Verification items for the finished model (mm, model axes). A direction names the side the tool comes from. Coordinates: 2 decimals unless noted, no trailing zeros. Order: outer loops, then holes, each group sorted by start corner. A loop starts at its lowest first (then second) coordinate and runs counter-clockwise, first axis right, second up. Notation, with made-up numbers: M 11.25,-38 L 61.25,-38 A31 ccw 61.25,-13 Z; hole C -32,-10 d9. An arc over 180 degrees is marked long. Return JSON: item names as keys, results as strings. Group by question number.
1. Section check C-C, the plane x = 0.5. Record the cut outline in (y, z).
2. Section check A-A, the plane x = 6. Record the cut outline in (y, z), plus the area to 3 significant figures.
3. Section check B-B, the plane z = 2.3. Give the number of separate pieces and of enclosed holes in the cut face, plus the area to 3 significant figures.
4. Set-up check for faces 1 (the flat face through (-8, 12.5, 1)), 2 (the flat face through (0, 4, 0)): record each of +Z, -Z, +X, -X, +Y, -Y from which the full face is reachable in a straight line by a thin tool's end or side.
5. Mould release check, pull along Y, two halves, no side actions. Record for faces 3 (the flat face through (5.96, 11.604, 1.479)), 4 (the flat face through (0, 15, 1)), 5 (the flat face through (0, 4, 3)): +Y half, -Y half, draft (parallel to the pull), parting line (faces both ways), or undercut.
6. Material ranges on line 1 along Y through (x, z) = (-6.75, 2.7); line 2 along Y through (x, z) = (6.5, 2.65); line 3 along X through (y, z) = (5.5, 0.4), recorded low to high.
```python
from build123d import *

# Parameters (mm, degrees)
SALIENTE_EXTRUIR3_DEPTH = 3


with BuildPart() as part:
    # Croquis1 → Saliente-Extruir3 (new body)
    with BuildSketch(Plane.XY):
        Polygon((-11.260603559, 15), (-15, 15), (-15, 3.468631071), (-15, -2.593220906), (-15, -15), (15, -15), (15, 15), (10.926682634, 15), (5.464101822, 15), (-4.343979365, 15), align=None)
        Polygon((-4.598156154, -12.5), (-10.987751023, -12.5), (-9.843926146, -10.486593018), (-5.795898544, -10.458408789), align=None, mode=Mode.SUBTRACT)
        Polygon((-1.735474056, -6.470030855), (1.725204311, -6.464101615), (3.460678367, -9.458172375), (2.574022478, -11), (1.788213156, -12.366463064), (1.735474056, -12.458172375), (1.711420323, -12.5), (-1.70439628, -12.5), (-1.725204311, -12.464101615), (-2.573851712, -11), (-3.460678367, -9.470030855), align=None, mode=Mode.SUBTRACT)
        Polygon((-9.52712635, -7.980422404), (-11, -5.43688968), (-11.262605478, -4.983391428), (-11, -4.527191603), (-9.53484008, -1.981906927), (-6.071595554, -1.977453403), (-4.336116426, -4.974484379), (-6.063881824, -7.97596888), align=None, mode=Mode.SUBTRACT)
        Polygon((10.94791539, -12.5), (5.442868782, -12.5), (6.463594896, -10.732050867), (9.927189585, -10.732050867), align=None, mode=Mode.SUBTRACT)
        Polygon((2, 3.464101615), (4, 0), (2, -3.464101615), (-2, -3.464101615), (-4, 0), (-2, 3.464101615), align=None, mode=Mode.SUBTRACT)
        Polygon((9.928710122, -1.732928769), (10.635389239, -2.957649744), (11, -3.589543959), (11.659747147, -4.732928769), (11, -5.874975703), (10.463594724, -6.803513255), (9.927189448, -7.732050808), (6.463594724, -7.731172846), (4.732557699, -4.731172846), (5.598456213, -3.232270202), (6.465115398, -1.732050808), align=None, mode=Mode.SUBTRACT)
        Polygon((-12.064918104, 0.484419433), (-12.5, -0.297648548), (-12.5, 1.211047664), align=None, mode=Mode.SUBTRACT)
        Polygon((-9.52712635, 7.980422404), (-6.063881824, 7.97596888), (-4.336116426, 4.974484379), (-6.071595554, 1.977453403), (-9.53484008, 1.981906927), (-10.26742004, 3.254549265), (-10.460255366, 3.589543959), (-10.62999033, 3.884408567), (-11, 4.527191603), (-11.262605478, 4.983391428), (-11, 5.43688968), (-10.401742938, 6.470030855), align=None, mode=Mode.SUBTRACT)
        Polygon((-9.843926146, 10.486593018), (-10.987751023, 12.5), (-4.598156154, 12.5), (-5.795898544, 10.458408789), align=None, mode=Mode.SUBTRACT)
        Polygon((1.725204311, 12.5), (2.604960918, 11), (3.49176728, 9.487980048), (1.766562969, 6.452081663), (-1.725204311, 6.42820323), (-3.49176728, 9.440223182), (-2.605395818, 11), (-1.766562969, 12.476121567), align=None, mode=Mode.SUBTRACT)
        Polygon((12.5, 1.211047664), (12.5, -0.297648548), (12.064918104, 0.484419433), align=None, mode=Mode.SUBTRACT)
        Polygon((11, 3.589543959), (9.928710122, 1.732928769), (6.465115398, 1.732050808), (4.732557699, 4.731172846), (6.463594724, 7.731172846), (9.927189448, 7.732050808), (11, 5.874975703), (11.659747147, 4.732928769), align=None, mode=Mode.SUBTRACT)
        Polygon((6.463594896, 10.732050808), (5.442868954, 12.5), (10.947915528, 12.5), (9.927189585, 10.732050808), align=None, mode=Mode.SUBTRACT)
    extrude(amount=SALIENTE_EXTRUIR3_DEPTH)


solid = part.part
```
Answers follow:
{
 "1": {"outline": "M -15,0 L -12.5,0 L -12.5,3 L -15,3 Z; M -6.47,0 L -3.46,0 L -3.46,3 L -6.47,3 Z; M 3.46,0 L 6.44,0 L 6.44,3 L 3.46,3 Z; M 12.49,0 L 15,0 L 15,3 L 12.49,3 Z"},
 "2": {"outline": "M -15,0 L -12.5,0 L -12.5,3 L -15,3 Z; M -11.54,0 L -6.93,0 L -6.93,3 L -11.54,3 Z; M -2.54,0 L 2.54,0 L 2.54,3 L -2.54,3 Z; M 6.93,0 L 11.54,0 L 11.54,3 L 6.93,3 Z; M 12.5,0 L 15,0 L 15,3 L 12.5,3 Z", "area": "57.9 mm^2"},
 "3": {"separate pieces": "1", "enclosed holes": "13", "area": "633 mm^2"},
 "4": {"face 1": "+Z, -Z", "face 2": "-Z, +X, -X, +Y, -Y"},
 "5": {"face 3": "undercut", "face 4": "+Y half", "face 5": "draft"},
 "6": {"line 1": "-15 to -12.5, -10.47 to -7.98, -1.98 to 1.98, 7.98 to 10.47, 12.5 to 15", "line 2": "-15 to -12.5, -10.73 to -7.73, -1.73 to 1.73, 7.73 to 10.73, 12.5 to 15", "line 3": "-15 to -10.96, -4.64 to 5.18, 11.22 to 15"}
}
